Geometry check sheet. Reference: the model listing, model coordinates, mm. Round coordinates to 2 decimals unless told otherwise and drop trailing zeros. Order: outer loops, then holes, each group sorted by start corner. A loop starts at its lowest first (then second) coordinate and runs counter-clockwise, first axis right, second up.
(1) Sectioned sample at C-C (x = -38.5). Record the boundary of the cut face in (y, z), plus the area to 3 significant figures.
(2) Sectioned sample at D-D (y = 1.75). Give the number of separate pieces and of enclosed holes in the cut face, plus the area to 3 significant figures.
(3) Sectioned sample at A-A (x = 0). Record the boundary of the cut face in (y, z).
(4) Sectioned sample at B-B (z = 0). Record the boundary of the cut face in (x, y), plus the area to 3 significant figures.
(5) Material ranges on line 1 along Z through (x, y) = (0, 2.75); line 2 along X through (y, z) = (4, -38.25); line 3 along Z through (x, y) = (39, 3.85), recorded low to high.
(6) Release check for a two-part mould opening along X. For faces 1 (the face through (-45, 2, 1)), 2 (the face through (-1, 2, -45)), 3 (the face through (15, 2, 0)) record: +X half, -X half, draft (parallel to the pull), parting line (faces both ways), or undercut.
from build123d import *

# Parameters (mm, degrees)
SKETCH1_W               = 90
SKETCH1_H               = 90
SKETCH1_R               = 2
BOSS_EXTRUDE1_DEPTH     = 5
SKETCH2_R               = 1.75
SKETCH2_W               = 5
SKETCH2_H               = 10
CUT_EXTRUDE1_DEPTH      = 1
CUT_EXTRUDE1_DEPTH_BACK = 6


with BuildPart() as part:
    # Sketch1 → Boss-Extrude1 (new body)
    with BuildSketch(Plane(origin=(0, 0, 0), x_dir=(1, 0, 0), z_dir=(0, 1, 0))):
        Rectangle(SKETCH1_W, SKETCH1_H)
        Circle(SKETCH1_R, mode=Mode.SUBTRACT)
        with BuildLine():
            Line((-26.585786438, 19.514718626), (-14.489985056, 7.418917244))
            ThreePointArc((-14.489985056, 7.418917244), (-13.949056578, 6.425915745), (-14.033116428, 5.298267955))
            ThreePointArc((-14.033116428, 5.298267955), (-15, 0), (-14.033116428, -5.298267955))
            ThreePointArc((-14.033116428, -5.298267955), (-13.949056578, -6.425915745), (-14.489985056, -7.418917244))
            Line((-14.489985056, -7.418917244), (-26.585786438, -19.514718626))
            ThreePointArc((-26.585786438, -19.514718626), (-28.765366865, -19.948264128), (-30, -18.100505063))
            Line((-30, -18.100505063), (-30, 18.100505063))
            ThreePointArc((-30, 18.100505063), (-28.765366865, 19.948264128), (-26.585786438, 19.514718626))
        make_face(mode=Mode.SUBTRACT)
        with BuildLine():
            Line((-18.100505063, 30), (18.100505063, 30))
            ThreePointArc((18.100505063, 30), (19.948264128, 28.765366865), (19.514718626, 26.585786438))
            Line((19.514718626, 26.585786438), (7.418917244, 14.489985056))
            ThreePointArc((7.418917244, 14.489985056), (6.425915745, 13.949056578), (5.298267955, 14.033116428))
            ThreePointArc((5.298267955, 14.033116428), (0, 15), (-5.298267955, 14.033116428))
            ThreePointArc((-5.298267955, 14.033116428), (-6.425915745, 13.949056578), (-7.418917244, 14.489985056))
            Line((-7.418917244, 14.489985056), (-19.514718626, 26.585786438))
            ThreePointArc((-19.514718626, 26.585786438), (-19.948264128, 28.765366865), (-18.100505063, 30))
        make_face(mode=Mode.SUBTRACT)
        with BuildLine():
            Line((30, 18.100505063), (30, -18.100505063))
            ThreePointArc((30, -18.100505063), (28.765366865, -19.948264128), (26.585786438, -19.514718626))
            Line((26.585786438, -19.514718626), (14.489985056, -7.418917244))
            ThreePointArc((14.489985056, -7.418917244), (13.949056578, -6.425915745), (14.033116428, -5.298267955))
            ThreePointArc((14.033116428, -5.298267955), (15, 0), (14.033116428, 5.298267955))
            ThreePointArc((14.033116428, 5.298267955), (13.949056578, 6.425915745), (14.489985056, 7.418917244))
            Line((14.489985056, 7.418917244), (26.585786438, 19.514718626))
            ThreePointArc((26.585786438, 19.514718626), (28.765366865, 19.948264128), (30, 18.100505063))
        make_face(mode=Mode.SUBTRACT)
        with BuildLine():
            Line((19.514718626, -26.585786438), (7.418917244, -14.489985056))
            ThreePointArc((7.418917244, -14.489985056), (6.425915745, -13.949056578), (5.298267955, -14.033116428))
            ThreePointArc((5.298267955, -14.033116428), (0, -15), (-5.298267955, -14.033116428))
            ThreePointArc((-5.298267955, -14.033116428), (-6.425915745, -13.949056578), (-7.418917244, -14.489985056))
            Line((-7.418917244, -14.489985056), (-19.514718626, -26.585786438))
            ThreePointArc((-19.514718626, -26.585786438), (-19.948264128, -28.765366865), (-18.100505063, -30))
            Line((-18.100505063, -30), (18.100505063, -30))
            ThreePointArc((18.100505063, -30), (19.948264128, -28.765366865), (19.514718626, -26.585786438))
        make_face(mode=Mode.SUBTRACT)
    extrude(amount=BOSS_EXTRUDE1_DEPTH)

    # Sketch2 → Cut-Extrude1 (cut, two sides)
    with BuildSketch(Plane(origin=(0, 5, 0), x_dir=(1, 0, 0), z_dir=(0, 1, 0))) as cut_extrude1_sk:
        with Locations((-30, -38.25)):
            Circle(SKETCH2_R)
        with Locations((30, -38.25)):
            Circle(SKETCH2_R)
        with Locations((30, 38.25)):
            Circle(SKETCH2_R)
        with Locations((-30, 38.25)):
            Circle(SKETCH2_R)
        with Locations((37.5, 25)):
            Rectangle(SKETCH2_W, SKETCH2_H)
        with Locations((37.5, -25)):
            Rectangle(SKETCH2_W, SKETCH2_H)
        with Locations((-37.5, -25)):
            Rectangle(SKETCH2_W, SKETCH2_H)
        with Locations((-37.5, 25)):
            Rectangle(SKETCH2_W, SKETCH2_H)
    extrude(amount=CUT_EXTRUDE1_DEPTH, mode=Mode.SUBTRACT)
    extrude(cut_extrude1_sk.sketch, amount=-CUT_EXTRUDE1_DEPTH_BACK, mode=Mode.SUBTRACT)


solid = part.part
Answer below:
1. outline: (0, -45) - (5, -45) - (5, -30) - (0, -30) - close; (0, -20) - (5, -20) - (5, 20) - (0, 20) - close; (0, 30) - (5, 30) - (5, 45) - (0, 45) - close
1. area: 350 mm2
2. separate pieces: 1
2. enclosed holes: 13
2. area: 6,010 mm2
3. outline: (0, -45) - (5, -45) - (5, -30) - (0, -30) - close; (0, -15) - (5, -15) - (5, -2) - (0, -2) - close; (0, 2) - (5, 2) - (5, 15) - (0, 15) - close; (0, 30) - (5, 30) - (5, 45) - (0, 45) - close
4. outline: (-45, 0) - (-30, 0) - (-30, 5) - (-45, 5) - close; (-15, 0) - (-2, 0) - (-2, 5) - (-15, 5) - close; (2, 0) - (15, 0) - (15, 5) - (2, 5) - close; (30, 0) - (45, 0) - (45, 5) - (30, 5) - close
4. area: 280 mm2
5. line 1: z = -45 to -30, -15 to -2, 2 to 15, 30 to 45
5. line 2: x = -45 to -31.75, -28.25 to 28.25, 31.75 to 45
5. line 3: z = -45 to -30, -20 to 20, 30 to 45
6. face 1: -X half
6. face 2: draft
6. face 3: undercut
